```python
from build123d import *

# Parameters (mm, degrees)
F1_DEPTH  = 6.35
F3_D      = 6.35
F5_D      = 6.35
F8_D      = 6.35
F10_D     = 6.35
F11_W     = 7.62
F11_H     = 10.5918
F12_DEPTH = 25.4


with BuildPart() as f1:
    # F0 (on Top) → F1 (new body)
    with BuildSketch(Plane.XY):
        Polygon((-279.4, 228.631461), (-279.4, -241.268539), (279.4, -241.268539), (279.4, 228.631461), (152.4, 228.631461), (152.4, 190.531461), (-152.4, 190.531461), (-152.4, 228.631461), align=None)
    extrude(amount=F1_DEPTH)

    # F3 (through all)
    with Locations(Plane.XY.offset(6.35)):
        with Locations((-234.68838, -189.198539), (-184.42432, -189.198539)):
            Hole(F3_D / 2)

    # F5 (through all)
    with Locations(Plane.XY.offset(6.35)):
        with Locations((-234.696, -67.278539), (-184.4294, -67.278539), (-184.4294, -107.918539), (-234.696, -107.918539), (-234.696, -148.558539), (-184.43194, -148.558539)):
            Hole(F5_D / 2)

    # F8 (through all)
    with Locations(Plane.XY.offset(6.35)):
        with Locations((184.404, -189.198539), (234.66806, -189.198539), (234.696, -148.558539), (184.43194, -148.558539), (184.4294, -107.918539), (234.696, -107.918539), (234.696, -67.278539), (184.43194, -67.278539)):
            Hole(F8_D / 2)

    # F10 (through all)
    with Locations(Plane.XY.offset(6.35)):
        with Locations((-52.07, 182.27294), (52.07, 182.27294), (52.07, 0), (-52.07, 0)):
            Hole(F10_D / 2)

    # F11 (on face) → F12 (cut)
    with BuildSketch(Plane.XY.offset(6.35)):
        with Locations((104.4448, 57.829161)):
            Rectangle(F11_W, F11_H)
        with Locations((104.23652, 159.429161)):
            Rectangle(F11_W, F11_H)
        with Locations((237.41888, 159.429161)):
            Rectangle(F11_W, F11_H)
        with Locations((237.2106, 57.829161)):
            Rectangle(F11_W, F11_H)
    extrude(amount=-F12_DEPTH, mode=Mode.SUBTRACT)


solid = f1.part
```
Source: CAD feature listing. Evaluate the final solid. Frame: model axes, mm. Round coordinates to 2 decimals unless told otherwise and drop trailing zeros. Write each loop counter-clockwise with the first axis right and the second up, starting at its lowest first coordinate (ties: lowest second). Pieces come first, ordered by that corner, then holes. Notation, with made-up numbers: M 78.25,30.25 L 87.25,30.25 A7 ccw 87.25,43.25 Z; hole C -26,-17.5 d6. An arc over 180 degrees is marked long. Answer as a JSON object with one key per item and string values. Group by question number.
(1) Section query A-A on x = -132. Output: boundary loops of the cut face in (y, z).
(2) Section query B-B on z = 2.5. State how many separate pieces and enclosed holes the cut face has, then the cut area to 3 significant figures.
(3) First-contact query: pin 1 (5 mm diameter, centred on x = -52.07, y = 182.27, fed in from +Z); pin 2 (2 mm diameter, centred on x = 1.5, z = 5, fed in from +Y). Flat tips, straight axial feed; report the tip coordinate or a pass-through.
(4) Ray query, line 1 (X direction, y = -110, z = 6); line 2 (X direction, y = 185, z = 4); line 3 (Y direction, x = 116, z = 3.5). Return the intervals inside material, ascending. Write a range as [from, to].
Computed values:
{
 "1": {"outline": "M -241.27,0 L 190.53,0 L 190.53,6.35 L -241.27,6.35 Z"},
 "2": {"separate pieces": "1", "enclosed holes": "24", "area": "250,000 mm^2"},
 "3": {"pin 1": "through", "pin 2": "y = 190.53"},
 "4": {"line 1": "[-279.4, -237.09], [-232.3, -186.83], [-182.03, 182.03], [186.83, 232.3], [237.09, 279.4]", "line 2": "[-279.4, -53.7], [-50.44, 50.44], [53.7, 279.4]", "line 3": "[-241.27, 190.53]"}
}
